Here's how the part is built. I have some questions about the finished solid (model axes, mm). Face numbers are marked on the shaded views. A direction names the side the tool comes from. Coordinates: 2 decimals unless noted, no trailing zeros. Write each loop counter-clockwise with the first axis right and the second up, starting at its lowest first coordinate (ties: lowest second). Pieces come first, ordered by that corner, then holes. Notation, with made-up numbers: (72.25, 49) - (100.25, 49) arc R17 ccw to (100.25, 60) - close; hole circle Ø5 at (-17, -29). An arc over 180 degrees is marked (long way). Answer in a Markdown table with one row per item. Add a question column.
Item 1: Imagine slicing it at B-B (y = -24.53). Please give me the cut outline in (x, z), plus the area to 3 significant figures.
Item 2: If I drill on probe 1 along X at (y, z) = (-23, -67.5); probe 2 along Z at (x, y) = (16.2, -24.53); probe 3 along X at (y, z) = (-26, -72.5), over which ranges is the centre line in solid material (lowest first)? Write a range as from..to.
Item 3: Which directions (+Z, -Z, +X, -X, +Y, -Y) give clear straight access to the entire face, cutting with the end or side of a thin tool? Please do the marked faces 1 and 2.
Item 4: Imagine slicing it at A-A (x = 16). State how many separate pieces and enclosed holes the cut face has, plus the area to 3 significant figures.
Item 5: We'd pull the mould along Z, two halves only. Please class the marked faces 3, 4 and 5: +Z half, -Z half, draft (parallel to the pull), parting line (faces both ways), or undercut.
Item 6: I'm going to push flat-ended pins straight in: pin 1 (1.4 mm diameter, centred on x = -14.5, y = -23.5, fed in from -Z); pin 2 (0.8 mm diameter, centred on x = 16, y = -25, fed in from -Z). Where does each tip first touch, or does it pass through?
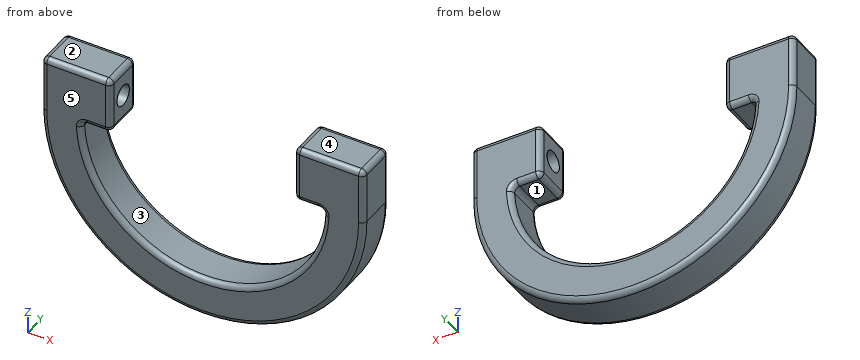
from build123d import *

# Parameters (mm, degrees)
BOSS_EXTRU_1_DEPTH      = 6
CONG_1_R                = 0.75
ESQUISSE2_R             = 1.5
ENL_V_MAT_EXTRU_1_DEPTH = 6
ENL_V_START             = -6
ESQUISSE3_R             = 1.5
ENL_V_MAT_EXTRU_2_DEPTH = 6


with BuildPart() as part:
    # Esquisse1 → Boss.-Extru.1 (new body)
    with BuildSketch(Plane(origin=(0, -27.53, 0), x_dir=(-1, 0, 0), z_dir=(0, 1, 0))):
        with BuildLine():
            Line((-23.997779507, -61.133700741), (-13.997779507, -61.133700741))
            Line((-13.997779507, -61.133700741), (-13.997779507, -69.133700741))
            Line((-13.997779507, -69.133700741), (-18.247779507, -69.133700741))
            ThreePointArc((-18.247779507, -69.133700741), (-0.747779507, -86.633700741), (16.752220493, -69.133700741))
            Line((16.752220493, -69.133700741), (12.502220493, -69.133700741))
            Line((12.502220493, -69.133700741), (12.502220493, -61.133700741))
            Line((12.502220493, -61.133700741), (22.502220493, -61.133700741))
            Line((22.502220493, -61.133700741), (22.502220493, -69.133700741))
            ThreePointArc((22.502220493, -69.133700741), (-0.747779507, -92.383700741), (-23.997779507, -69.133700741))
            Line((-23.997779507, -69.133700741), (-23.997779507, -61.133700741))
        make_face()
    extrude(amount=BOSS_EXTRU_1_DEPTH)

    # Congé1
    cong_1_edges = [part.edges().sort_by_distance(p)[0] for p in [
        (23.997779507, -21.53, -65.133700741),
        (-14.627220493, -27.53, -69.133700741),
        (-12.502220493, -27.53, -65.133700741),
        (-17.502220493, -27.53, -61.133700741),
        (-22.502220493, -27.53, -65.133700741),
        (0.747779507, -27.53, -92.383700741),
        (23.997779507, -27.53, -65.133700741),
        (18.997779507, -27.53, -61.133700741),
        (13.997779507, -27.53, -65.133700741),
        (0.747779507, -21.53, -92.383700741),
        (-22.502220493, -21.53, -65.133700741),
        (13.997779507, -24.53, -69.133700741),
        (18.247779507, -24.53, -69.133700741),
        (-16.752220493, -24.53, -69.133700741),
        (-12.502220493, -24.53, -69.133700741),
        (-12.502220493, -24.53, -61.133700741),
        (-22.502220493, -24.53, -61.133700741),
        (23.997779507, -24.53, -61.133700741),
        (13.997779507, -24.53, -61.133700741),
        (-17.502220493, -21.53, -61.133700741),
        (-12.502220493, -21.53, -65.133700741),
        (-14.627220493, -21.53, -69.133700741),
        (0.747779507, -21.53, -86.633700741),
        (16.122779507, -21.53, -69.133700741),
        (13.997779507, -21.53, -65.133700741),
        (18.997779507, -21.53, -61.133700741),
        (16.122779507, -27.53, -69.133700741),
        (0.747779507, -27.53, -86.633700741),
    ]]
    fillet(cong_1_edges, radius=CONG_1_R)

    # Esquisse2 → Enlèv. mat.-Extru.1 (cut)
    with BuildSketch(Plane(origin=(-12.502220493, 0, 0), x_dir=(0, 0, -1), z_dir=(1, 0, 0))):
        with Locations((65.133700741, -24.53)):
            Circle(ESQUISSE2_R)
    extrude(amount=-ENL_V_MAT_EXTRU_1_DEPTH, mode=Mode.SUBTRACT)

    # Esquisse3 → Enlèv. mat.-Extru.2 (cut)
    with BuildSketch(Plane.ZY.offset(-13.997779507).offset(ENL_V_START)):
        with Locations(Location((-65.133700741, -24.53, 0), (0, 0, 180))):
            Circle(ESQUISSE3_R)
    extrude(amount=ENL_V_MAT_EXTRU_2_DEPTH, mode=Mode.SUBTRACT)


solid = part.part
Here are the results:
| question | item | result |
|---|---|---|
| 1 | outline | (-22.5, -69.13) arc R23.25 ccw to (24, -69.13) - (24, -61.88) arc R0.75 ccw to (23.25, -61.13) - (14.75, -61.13) arc R0.75 ccw to (14, -61.88) - (14, -63.63) - (20, -63.63) - (20, -66.63) - (14, -66.63) - (14, -68.38) arc R0.75 ccw to (14.75, -69.13) - (17.48, -69.13) arc R0.75 cw to (18.23, -69.92) arc R17.5 cw to (-16.73, -69.92) arc R0.75 cw to (-15.99, -69.13) - (-13.25, -69.13) arc R0.75 ccw to (-12.5, -68.38) - (-12.5, -66.63) - (-18.5, -66.63) - (-18.5, -63.63) - (-12.5, -63.63) - (-12.5, -61.88) arc R0.75 ccw to (-13.25, -61.13) - (-21.75, -61.13) arc R0.75 ccw to (-22.5, -61.88) - close |
| 1 | area | 492 mm2 |
| 2 | probe 1 | x = -22.5..-12.5, 14..24 |
| 2 | probe 2 | z = -86.51..-77.35, -69.13..-66.63, -63.63..-61.13 |
| 2 | probe 3 | x = -22.26..-16.43, 17.92..23.75 |
| 3 | face 1 | +Y, -Y |
| 3 | face 2 | +Z, +X, -X, +Y, -Y |
| 4 | separate pieces | 2 |
| 4 | enclosed holes | 1 |
| 4 | area | 93.5 mm2 |
| 5 | face 3 | undercut |
| 5 | face 4 | +Z half |
| 5 | face 5 | draft |
| 6 | pin 1 | stops at z = -87.27 |
| 6 | pin 2 | stops at z = -87.02 |
